Input: part model. Units: mm. Frame: model coordinates. Round coordinates to 2 decimals unless told otherwise and drop trailing zeros. Write each loop counter-clockwise with the first axis right and the second up, starting at its lowest first coordinate (ties: lowest second). Pieces come first, ordered by that corner, then holes. Notation, with made-up numbers: (-15, 40.5) -> (38, 40.5) arc R18 ccw to (38, 61.5) -> close; hole circle Ø9 at (8, 66.5). An arc over 180 degrees is marked (long way). Write item = value, one per line.
```python
from build123d import *

# Parameters (mm, degrees)
SALIENTE_EXTRUIR1_DEPTH = 0.1


with BuildPart() as part:
    # Model → Saliente-Extruir1 (new body)
    with BuildSketch(Plane.XY):
        with BuildLine():
            Line((83.956301506, -17.166999348), (84.015376633, -18.477240051))
            Line((84.015376633, -18.477240051), (85.336602283, -18.077638007))
            Line((85.336602283, -18.077638007), (84.538223467, -17.008293358))
            ThreePointArc((84.538223467, -17.008293358), (84.278969465, -16.042382101), (83.786477348, -15.171951914))
            ThreePointArc((83.786477348, -15.171951914), (83.576571308, -14.005422888), (83.198659759, -12.8820203))
            ThreePointArc((83.198659759, -12.8820203), (83.21653602, -12.153238047), (83.021147285, -11.450908798))
            ThreePointArc((83.021147285, -11.450908798), (83.091174716, -9.918606089), (82.654557847, -8.448156791))
            ThreePointArc((82.654557847, -8.448156791), (83.012265392, -6.298296984), (82.511107342, -4.177284848))
            ThreePointArc((82.511107342, -4.177284848), (82.63621748, -2.505599358), (82.234450021, -0.878095799))
            ThreePointArc((82.234450021, -0.878095799), (82.435913685, 0.460640045), (82.268030876, 1.804000246))
            ThreePointArc((82.268030876, 1.804000246), (82.996051805, 3.402356573), (82.865109648, 5.153816414))
            ThreePointArc((82.865109648, 5.153816414), (83.401985842, 6.694986621), (83.724308061, 8.294846004))
            ThreePointArc((83.724308061, 8.294846004), (85.978479306, 21.570456798), (86.584690484, 35.022432042))
            ThreePointArc((86.584690484, 35.022432042), (86.416684054, 39.135370857), (86.088155048, 43.23860867))
            ThreePointArc((86.088155048, 43.23860867), (84.060345255, 49.407216919), (79.615503089, 54.140832704))
            ThreePointArc((79.615503089, 54.140832704), (69.080555659, 59.249963441), (57.51663409, 61.084098716))
            ThreePointArc((57.51663409, 61.084098716), (45.952712521, 59.249963441), (35.417765091, 54.140832704))
            ThreePointArc((35.417765091, 54.140832704), (30.972922925, 49.407216919), (28.945113132, 43.23860867))
            ThreePointArc((28.945113132, 43.23860867), (28.46242928, 29.95974371), (29.654838805, 16.72571946))
            ThreePointArc((29.654838805, 16.72571946), (29.473058184, 11.615593771), (29.015376633, 6.522759949))
            ThreePointArc((29.015376633, 6.522759949), (28.442846773, 4.643578134), (28.610136964, 2.6862512))
            ThreePointArc((28.610136964, 2.6862512), (28.323722373, 0.618533481), (28.978689788, -1.363512826))
            ThreePointArc((28.978689788, -1.363512826), (28.890519119, -2.843965116), (29.162248311, -4.30193504))
            ThreePointArc((29.162248311, -4.30193504), (29.034928035, -5.947952582), (29.360669993, -7.566432232))
            ThreePointArc((29.360669993, -7.566432232), (29.77476773, -9.238513166), (30.644216328, -10.725587717))
            ThreePointArc((30.644216328, -10.725587717), (30.987352099, -11.946605577), (31.558807946, -13.078888662))
            ThreePointArc((31.558807946, -13.078888662), (31.963393581, -14.170963904), (32.606401809, -15.141972807))
            ThreePointArc((32.606401809, -15.141972807), (32.871834994, -15.95176655), (33.355447957, -16.653435407))
            Line((33.355447957, -16.653435407), (33.414523084, -17.96367611))
            Line((33.414523084, -17.96367611), (34.735748735, -17.564074065))
            Line((34.735748735, -17.564074065), (33.937369918, -16.494729417))
            ThreePointArc((33.937369918, -16.494729417), (33.678115916, -15.52881816), (33.185623799, -14.658387973))
            ThreePointArc((33.185623799, -14.658387973), (32.97571776, -13.491858947), (32.59780621, -12.368456359))
            ThreePointArc((32.59780621, -12.368456359), (32.615682471, -11.639674106), (32.420293737, -10.937344857))
            ThreePointArc((32.420293737, -10.937344857), (32.490321167, -9.405042148), (32.053704298, -7.93459285))
            ThreePointArc((32.053704298, -7.93459285), (32.411411843, -5.784733043), (31.910253793, -3.663720907))
            ThreePointArc((31.910253793, -3.663720907), (32.035363932, -1.992035417), (31.633596472, -0.364531858))
            ThreePointArc((31.633596472, -0.364531858), (31.835060136, 0.974203986), (31.667177327, 2.317564187))
            ThreePointArc((31.667177327, 2.317564187), (32.395198256, 3.915920514), (32.2642561, 5.667380355))
            ThreePointArc((32.2642561, 5.667380355), (33.036563223, 9.618087334), (34.015376633, 13.522759949))
            ThreePointArc((34.015376633, 13.522759949), (34.500457554, 15.949651286), (34.706334447, 18.41596833))
            ThreePointArc((34.706334447, 18.41596833), (31.522529085, 33.538428771), (33.337993753, 48.885399624))
            ThreePointArc((33.337993753, 48.885399624), (41.857208532, 49.214409123), (48.657173595, 54.356951572))
            ThreePointArc((48.657173595, 54.356951572), (65.042417717, 50.813818289), (81.695137016, 48.885876802))
            ThreePointArc((81.695137016, 48.885876802), (83.511455819, 33.554448429), (80.338345767, 18.445408666))
            ThreePointArc((80.338345767, 18.445408666), (80.983262934, 12.168889843), (79.616230182, 6.009196008))
            ThreePointArc((79.616230182, 6.009196008), (79.043700322, 4.130014193), (79.210990513, 2.172687259))
            ThreePointArc((79.210990513, 2.172687259), (78.924575921, 0.10496954), (79.579543337, -1.877076767))
            ThreePointArc((79.579543337, -1.877076767), (79.491372668, -3.357529058), (79.763101859, -4.815498981))
            ThreePointArc((79.763101859, -4.815498981), (79.635781584, -6.461516523), (79.961523541, -8.079996173))
            ThreePointArc((79.961523541, -8.079996173), (80.375621279, -9.752077107), (81.245069877, -11.239151658))
            ThreePointArc((81.245069877, -11.239151658), (81.588205648, -12.460169518), (82.159661495, -13.592452603))
            ThreePointArc((82.159661495, -13.592452603), (82.56424713, -14.684527845), (83.207255358, -15.655536748))
            ThreePointArc((83.207255358, -15.655536748), (83.472688543, -16.465330491), (83.956301506, -17.166999348))
        make_face()
    extrude(amount=SALIENTE_EXTRUIR1_DEPTH)


solid = part.part
```
1) Line query: L1, parallel to X at y = 11.5, z = 0.05; L2, parallel to Y at x = 56.5, z = 0.05; L3, parallel to Y at x = 78, z = 0.05. Output: solid intervals per line, ascending. Write a range as from..to.
Solutions:
L1 = 29.47..33.48, 80.93..84.42
L2 = 52.45..61.06
L3 = 49.17..55.19
2) Cut plane A-A (y = 11). Return the cut outline in (x, z).
Solutions:
outline = (29.43, 0) -> (33.36, 0) -> (33.36, 0.1) -> (29.43, 0.1) -> close; (80.88, 0) -> (84.32, 0) -> (84.32, 0.1) -> (80.88, 0.1) -> close
3) Cut plane D-D (x = 73). Return the cut outline in (y, z).
Solutions:
outline = (49.69, 0) -> (57.79, 0) -> (57.79, 0.1) -> (49.69, 0.1) -> close
4) Cut plane C-C (x = 59). Return the cut outline in (y, z).
Solutions:
outline = (51.93, 0) -> (61.04, 0) -> (61.04, 0.1) -> (51.93, 0.1) -> close
5) Cut plane B-B (y = 39). Return the cut outline in (x, z).
Solutions:
outline = (28.61, 0) -> (31.59, 0) -> (31.59, 0.1) -> (28.61, 0.1) -> close; (83.44, 0) -> (86.42, 0) -> (86.42, 0.1) -> (83.44, 0.1) -> close
